```python
from build123d import *

# Parameters (mm, degrees)
SKETCH_1_R          = 3.2
SKETCH_1_R_2        = 1.25
EXTRUDE_1_DEPTH     = 4.2
SKETCH_2_R          = 2.5
CUT_EXTRUDE_1_DEPTH = 3


with BuildPart() as part:
    # 스케치1 → 보스-돌출1 (new body)
    with BuildSketch(Plane.XY):
        Polygon((15, 24), (-15, 24), (-15, 18), (-30, 18), (-30, -18), (-15, -18), (-15, -24), (15, -24), (15, -18), (30, -18), (30, 18), (15, 18), align=None)
        with Locations((-25, 12.5)):
            Circle(SKETCH_1_R, mode=Mode.SUBTRACT)
        with Locations((-11, 20)):
            Circle(SKETCH_1_R_2, mode=Mode.SUBTRACT)
        with Locations((-11, -20)):
            Circle(SKETCH_1_R_2, mode=Mode.SUBTRACT)
        with Locations((-25, -12.5)):
            Circle(SKETCH_1_R, mode=Mode.SUBTRACT)
        with Locations((25, -12.5)):
            Circle(SKETCH_1_R, mode=Mode.SUBTRACT)
        with Locations((11, -20)):
            Circle(SKETCH_1_R_2, mode=Mode.SUBTRACT)
        with Locations((11, 20)):
            Circle(SKETCH_1_R_2, mode=Mode.SUBTRACT)
        with Locations((25, 12.5)):
            Circle(SKETCH_1_R, mode=Mode.SUBTRACT)
    extrude(amount=EXTRUDE_1_DEPTH)

    # 스케치2 → 컷-돌출1 (cut)
    with BuildSketch(Plane(origin=(0, 0, 0), x_dir=(-1, 0, 0), z_dir=(0, 0, -1))):
        with Locations((-11, 20)):
            Circle(SKETCH_2_R)
        with Locations((11, 20)):
            Circle(SKETCH_2_R)
        with Locations((11, -20)):
            Circle(SKETCH_2_R)
        with Locations((-11, -20)):
            Circle(SKETCH_2_R)
    extrude(amount=-CUT_EXTRUDE_1_DEPTH, mode=Mode.SUBTRACT)


solid = part.part
```
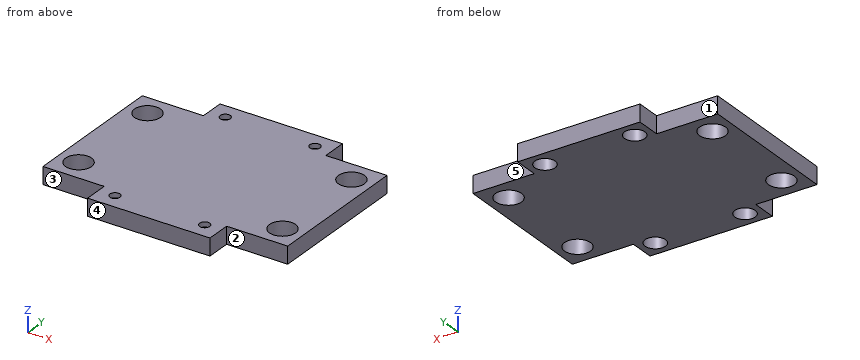
Verification items for the finished model (mm, model axes). Face numbers are marked on the shaded views. A direction names the side the tool comes from. Coordinates: 2 decimals unless noted, no trailing zeros. Loops run counter-clockwise (first coordinate to the right, second up) from the corner with the lowest first, then second, coordinate; pieces in that order, holes last. Notation, with made-up numbers: (-29.5, 44) -> (-22.5, 44) arc R22 ccw to (-22.5, 54) -> close; hole circle Ø7 at (75, 38.25). An arc over 180 degrees is marked (long way). Answer in a Markdown table with one row per item.
1) Section check D-D (x = -11). Record the cut outline in (y, z), and give its area (3 significant figures).
The answers:
| item | result |
|---|---|
| outline | (-24, 0) -> (-22.5, 0) -> (-22.5, 3) -> (-21.25, 3) -> (-21.25, 4.2) -> (-24, 4.2) -> close; (-18.75, 3) -> (-17.5, 3) -> (-17.5, 0) -> (17.5, 0) -> (17.5, 3) -> (18.75, 3) -> (18.75, 4.2) -> (-18.75, 4.2) -> close; (21.25, 3) -> (22.5, 3) -> (22.5, 0) -> (24, 0) -> (24, 4.2) -> (21.25, 4.2) -> close |
| area | 166 mm2 |
2) Access from +Z, -Z, +X, -X, +Y, -Y to the whole of each face (thin tool, end or side, straight path). Record for the marked faces 1, 2, 3, 4 and 5.
The answers:
| item | result |
|---|---|
| face 1 | +Z, -Z, -X, +Y |
| face 2 | +Z, -Z, +X, -Y |
| face 3 | +Z, -Z, -X, -Y |
| face 4 | +Z, -Z, +X, -X, -Y |
| face 5 | +Z, -Z, +X, +Y |
3) Section check A-A (x = 25). Record the cut outline in (y, z).
The answers:
| item | result |
|---|---|
| outline | (-18, 0) -> (-15.7, 0) -> (-15.7, 4.2) -> (-18, 4.2) -> close; (-9.3, 0) -> (9.3, 0) -> (9.3, 4.2) -> (-9.3, 4.2) -> close; (15.7, 0) -> (18, 0) -> (18, 4.2) -> (15.7, 4.2) -> close |
4) Depth check by flat-ended pin: P1, Ø10, axis at x = 25, y = 12.5, coming from the -Z side; P2, Ø3, axis at x = -11, y = 20, coming from the -Z side; P3, Ø1.3, axis at y = -21, z = 3, coming from the +X side; P4, Ø1, axis at x = 23, z = 2.5, coming from the -Y side. Enter the tip coordinate at first touch or a pass-through.
The answers:
| item | result |
|---|---|
| P1 | stops at z = 0 |
| P2 | stops at z = 3 |
| P3 | stops at x = 15 |
| P4 | stops at y = -18 |
5) Section check B-B (y = 20). Record the cut outline in (x, z), and give its area (3 significant figures).
The answers:
| item | result |
|---|---|
| outline | (-15, 0) -> (-13.5, 0) -> (-13.5, 3) -> (-12.25, 3) -> (-12.25, 4.2) -> (-15, 4.2) -> close; (-9.75, 3) -> (-8.5, 3) -> (-8.5, 0) -> (8.5, 0) -> (8.5, 3) -> (9.75, 3) -> (9.75, 4.2) -> (-9.75, 4.2) -> close; (12.25, 3) -> (13.5, 3) -> (13.5, 0) -> (15, 0) -> (15, 4.2) -> (12.25, 4.2) -> close |
| area | 90.0 mm2 |
6) Section check C-C (z = 2.3). Give the number of separate pieces and of enclosed holes in the cut face, and give its area (3 significant figures).
The answers:
| item | result |
|---|---|
| separate pieces | 1 |
| enclosed holes | 8 |
| area | 2,310 mm2 |
7) Scan lines: line 1 along Y through (x, z) = (11, 2); line 2 along Y through (x, z) = (25, 2.6); line 3 along X through (y, z) = (20, 3.85). Record each from-to range of solid material in increasing order. Write a range as from..to.
The answers:
| item | result |
|---|---|
| line 1 | y = -24..-22.5, -17.5..17.5, 22.5..24 |
| line 2 | y = -18..-15.7, -9.3..9.3, 15.7..18 |
| line 3 | x = -15..-12.25, -9.75..9.75, 12.25..15 |
